```python
from build123d import *

# Parameters (mm, degrees)
BOSS_EXTRUDE1_DEPTH     = 2
SKETCH3_W               = 3
SKETCH3_H               = 10
BOSS_EXTRUDE2_DEPTH     = 20
SKETCH4_R               = 2
CUT_EXTRUDE2_DEPTH      = 259.984555524
FILLET1_R               = 4
FILLET1_OF_MIRROR1_R    = 4
SKETCH5_R               = 2
CUT_EXTRUDE3_DEPTH      = 242.246761636
CUT_EXTRUDE4_DEPTH      = 242.420794465
CUT_EXTRUDE4_DEPTH_BACK = 242.420794465
SKETCH6_R               = 2
SKETCH7_W               = 32
SKETCH7_H               = 2
BOSS_EXTRUDE3_DEPTH     = 45
FILLET3_R               = 5
FILLET4_R               = 5
SKETCH8_R               = 2
CUT_EXTRUDE5_DEPTH      = 231.076617673


with BuildPart() as part:
    # Sketch1 → Boss-Extrude1 (new body)
    with BuildSketch(Plane(origin=(0, 0, 0), x_dir=(1, 0, 0), z_dir=(0, 1, 0))):
        with BuildLine():
            Line((70, -27.5), (70, -37.5))
            Line((70, -37.5), (50, -37.5))
            Line((50, -37.5), (50, -107.5))
            Line((50, -107.5), (70, -107.5))
            Line((70, -107.5), (70, -122.5))
            Line((70, -122.5), (50, -122.5))
            Line((50, -122.5), (50, -192.5))
            Line((50, -192.5), (70, -192.5))
            Line((70, -192.5), (70, -202.5))
            ThreePointArc((70, -202.5), (0, -230), (-70, -202.5))
            Line((-70, -202.5), (-70, -192.5))
            Line((-70, -192.5), (-50, -192.5))
            Line((-50, -192.5), (-50, -122.5))
            Line((-50, -122.5), (-70, -122.5))
            Line((-70, -122.5), (-70, -107.5))
            Line((-70, -107.5), (-50, -107.5))
            Line((-50, -107.5), (-50, -37.5))
            Line((-50, -37.5), (-70, -37.5))
            Line((-70, -37.5), (-70, -27.5))
            ThreePointArc((-70, -27.5), (0, 0), (70, -27.5))
        make_face()
    extrude(amount=BOSS_EXTRUDE1_DEPTH)

    # Sketch3 → Boss-Extrude2 (add)
    with BuildSketch(Plane(origin=(0, 2, 0), x_dir=(1, 0, 0), z_dir=(0, 1, 0))):
        with Locations((48.5, -157.5)):
            Rectangle(SKETCH3_W, SKETCH3_H)
    boss_extrude2 = extrude(amount=BOSS_EXTRUDE2_DEPTH)

    # Sketch4 → Cut-Extrude2 (cut, through all)
    with BuildSketch(Plane.ZY.offset(-47)):
        with Locations((157.5, 17)):
            Circle(SKETCH4_R)
    cut_extrude2 = extrude(amount=-CUT_EXTRUDE2_DEPTH, mode=Mode.SUBTRACT)

    # Fillet1
    fillet1_edges = [part.edges().sort_by_distance(p)[0] for p in [
        (47, 2, 157.5),
        (48.5, 2, 162.5),
        (48.5, 2, 152.5),
        (48.5, 22, 162.5),
        (48.5, 22, 152.5),
    ]]
    fillet(fillet1_edges, radius=FILLET1_R)

    # Mirror1: Boss-Extrude2, Cut-Extrude2 across plane
    add(boss_extrude2.mirror(Plane(origin=(0, 0, 0), x_dir=(0, 0, 1), z_dir=(1, 0, 0))))
    add(cut_extrude2.mirror(Plane(origin=(0, 0, 0), x_dir=(0, 0, 1), z_dir=(1, 0, 0))), mode=Mode.SUBTRACT)

    # Fillet1 of Mirror1
    fillet1_of_mirror1_edges = [part.edges().sort_by_distance(p)[0] for p in [
        (-47, 2, 157.5),
        (-48.5, 2, 162.5),
        (-48.5, 2, 152.5),
        (-48.5, 22, 162.5),
        (-48.5, 22, 152.5),
    ]]
    fillet(fillet1_of_mirror1_edges, radius=FILLET1_OF_MIRROR1_R)

    # Sketch5 → Cut-Extrude3 (cut, through all)
    with BuildSketch(Plane(origin=(0, 2, 0), x_dir=(1, 0, 0), z_dir=(0, 1, 0))):
        with Locations(Location((-60, -115, 0), (0, 0, 270))):
            Circle(SKETCH5_R)
        with Locations(Location((-60, -200.3, 0), (0, 0, 270))):
            Circle(SKETCH5_R)
        with Locations(Location((-60, -29.7, 0), (0, 0, 270))):
            Circle(SKETCH5_R)
        with Locations(Location((60, -200.3, 0), (0, 0, 90))):
            Circle(SKETCH5_R)
        with Locations(Location((60, -115, 0), (0, 0, 90))):
            Circle(SKETCH5_R)
        with Locations(Location((60, -29.7, 0), (0, 0, 90))):
            Circle(SKETCH5_R)
    extrude(amount=-CUT_EXTRUDE3_DEPTH, mode=Mode.SUBTRACT)

    # Sketch6 → Cut-Extrude4 (cut, two sides: drawn at the far end of the back side and taken through both)
    with BuildSketch(Plane.XZ.offset(-CUT_EXTRUDE4_DEPTH_BACK)):
        with Locations(Location((-27, 152.5, 0), (0, 0, 270))):
            Circle(SKETCH6_R)
        with Locations(Location((27, 152.5, 0), (0, 0, 270))):
            Circle(SKETCH6_R)
        with Locations(Location((-27, 113.5, 0), (0, 0, 270))):
            Circle(SKETCH6_R)
        with Locations(Location((27, 113.5, 0), (0, 0, 270))):
            Circle(SKETCH6_R)
    extrude(amount=CUT_EXTRUDE4_DEPTH + CUT_EXTRUDE4_DEPTH_BACK, mode=Mode.SUBTRACT)

    # Sketch7 → Boss-Extrude3 (add)
    with BuildSketch(Plane.XZ):
        with Locations((0, 213.5)):
            Rectangle(SKETCH7_W, SKETCH7_H)
    extrude(amount=BOSS_EXTRUDE3_DEPTH)

    # Fillet3
    fillet3_edges = [part.edges().sort_by_distance(p)[0] for p in [
        (-16, 0, 213.5),
        (16, 0, 213.5),
        (-16, -45, 213.5),
        (16, -45, 213.5),
    ]]
    fillet(fillet3_edges, radius=FILLET3_R)

    # Fillet4
    fillet4_edges = [part.edges().sort_by_distance(p)[0] for p in [
        (0, 0, 212.5),
    ]]
    fillet(fillet4_edges, radius=FILLET4_R)

    # Sketch8 → Cut-Extrude5 (cut, through all)
    with BuildSketch(Plane.XY.offset(214.5)):
        with Locations((-10.5, -19.5)):
            Circle(SKETCH8_R)
        with Locations((10.5, -19.5)):
            Circle(SKETCH8_R)
        with Locations((10.5, -32)):
            Circle(SKETCH8_R)
        with Locations((-10.5, -32)):
            Circle(SKETCH8_R)
    extrude(amount=-CUT_EXTRUDE5_DEPTH, mode=Mode.SUBTRACT)


solid = part.part
```
Geometry: final body of the model. Coordinates: model frame, mm. A direction names the side the tool comes from. Give positions to 0.01 mm unless a question says otherwise; leave off trailing zeros. Order: outer loops, then holes, each group sorted by start corner. A loop starts at its lowest first (then second) coordinate and runs counter-clockwise, first axis right, second up. Notation, with made-up numbers: (57.25, 55.25) -> (84.25, 55.25) arc R12 cw to (84.25, 69.25) -> close; hole circle Ø3 at (56.25, 19.5). An arc over 180 degrees is marked (long way). Write each question's results on one line, items separated by ' | '. Start each with the question number.
1) Section B-B (z = 141). Return loops of the section in (x, y).
2) Line query: line 1 (X direction, y = 0.85, z = 200.3); line 2 (Z direction, x = -47.75, y = 17); line 3 (Z direction, x = 60, y = 0.7). Output: solid intervals per line, ascending. Write a range as from..to.
3) Set-up query: faces 5 (the flat face through (0, -22, 214.5)), 6 (the flat face through (0, -25, 212.5)), 7 (the flat face through (-47, 14, 158)), 8 (the flat face through (50, 6, 157)). Return all of +Z, -Z, +X, -X, +Y, -Y with unobstructed straight access to the full face (end or side cutting, diameter ignored); none if empty.
4) First-contact query: pin 1 (2 mm diameter, centred on x = 42.5, z = 74.5, fed in from -Y); pin 2 (11 mm diameter, centred on y = 7, z = 143, fed in from +X); pin 3 (3 mm diameter, centred on x = 60, z = 200.3, fed in from -Y); pin 4 (8 mm diameter, centred on y = 11, z = 159.5, fed in from -X). Flat tips, straight axial feed; report the tip coordinate or a pass-through.
5) Draft query along X for faces 1 (the cylindrical face through (18, -1, 213)), 2 (the cylindrical face through (-1.078, 0.986, 0.006)), 3 (the flat face through (-50, 6, 158)), 4 (the flat face through (47, 14, 158)). Return one class per face: pulls with the +X half, pulls with the -X half, needs draft (parallel to the pull), parting line crosses it, or undercut.
6) Section A-A (x = 4). Return loops of the section in (y, z).
7) Section C-C (y = -11). Return loops of the section in (x, z).
Calculated:
1) outline: (-50, 0) -> (50, 0) -> (50, 2) -> (-50, 2) -> close
2) line 1: -70..-62, -58..58, 62..70 | line 2: 152.5..155.5, 159.5..162.5 | line 3: 19.32..27.7, 31.7..37.5, 107.5..113, 117..122.5, 192.5..198.3, 202.3..210.68
3) face 5: +Z, +X, -X, -Y | face 6: -Z, +X, -X, -Y | face 7: +Z, -Z, +Y | face 8: +X, +Y, -Y
4) pin 1: y = 0 | pin 2: x = 50 | pin 3: through | pin 4: x = -50
5) face 1: pulls with the +X half | face 2: parting line crosses it | face 3: pulls with the -X half | face 4: undercut
6) outline: (-45, 212.5) -> (-5, 212.5) arc R5 cw to (0, 207.5) -> (0, 0.08) -> (2, 0.08) -> (2, 229.92) -> (0, 229.92) -> (0, 214.5) -> (-45, 214.5) -> close
7) outline: (-16, 212.5) -> (16, 212.5) -> (16, 214.5) -> (-16, 214.5) -> close
